from build123d import *

# Parameters (mm, degrees)
SKETCH1_W           = 45
SKETCH1_H           = 187
SKETCH1_R           = 2.2
SKETCH1_R_2         = 2.075
BOSS_EXTRUDE1_DEPTH = 4.75
BOSS_EXTRUDE2_START = -15
SKETCH1_3_R         = 2.075
SKETCH1_3_W         = 2
SKETCH1_3_H         = 171
SKETCH1_3_W_2       = 3
BOSS_EXTRUDE2_DEPTH = 15


with BuildPart() as part:
    # Sketch1 → Boss-Extrude1 (new body)
    with BuildSketch(Plane.XY):
        with Locations((8, 0)):
            Rectangle(SKETCH1_W, SKETCH1_H)
        with Locations((0, -75.75)):
            Circle(SKETCH1_R, mode=Mode.SUBTRACT)
        with Locations((16, -75.75)):
            Circle(SKETCH1_R, mode=Mode.SUBTRACT)
        with Locations((0, 75.75)):
            Circle(SKETCH1_R, mode=Mode.SUBTRACT)
        with Locations((16, 75.75)):
            Circle(SKETCH1_R, mode=Mode.SUBTRACT)
        with Locations((8, -89.5)):
            Circle(SKETCH1_R_2, mode=Mode.SUBTRACT)
        with Locations(Location((8, 89.5, 0), (0, 0, 180))):
            Circle(SKETCH1_R_2, mode=Mode.SUBTRACT)
    extrude(amount=BOSS_EXTRUDE1_DEPTH)

    # Sketch1<3> → Boss-Extrude2 (add)
    # profile 1 of 5: a face of its own
    with BuildSketch(Plane.XY.offset(BOSS_EXTRUDE2_START)):
        Polygon((-12.5, 85.5), (-6.5, 85.5), (6.5, 85.5), (9.5, 85.5), (22.5, 85.5), (28.5, 85.5), (30.5, 85.5), (30.5, 93.5), (-14.5, 93.5), (-14.5, 85.5), align=None)
        with Locations(Location((8, 89.5, 0), (0, 0, 180))):
            Circle(SKETCH1_3_R, mode=Mode.SUBTRACT)
    # profile 2 of 5: a face of its own
    with BuildSketch(Plane.XY.offset(BOSS_EXTRUDE2_START)):
        with Locations((-13.5, 0)):
            Rectangle(SKETCH1_3_W, SKETCH1_3_H)
    # profile 3 of 5: a face of its own
    with BuildSketch(Plane.XY.offset(BOSS_EXTRUDE2_START)):
        Polygon((6.5, -85.5), (-6.5, -85.5), (-12.5, -85.5), (-14.5, -85.5), (-14.5, -93.5), (30.5, -93.5), (30.5, -85.5), (28.5, -85.5), (22.5, -85.5), (9.5, -85.5), align=None)
        with Locations(Location((8, -89.5, 0), (0, 0, 270))):
            Circle(SKETCH1_3_R, mode=Mode.SUBTRACT)
    # profile 4 of 5: a face of its own
    with BuildSketch(Plane.XY.offset(BOSS_EXTRUDE2_START)):
        with Locations((29.5, 0)):
            Rectangle(SKETCH1_3_W, SKETCH1_3_H)
    # profile 5 of 5: a face of its own
    with BuildSketch(Plane.XY.offset(BOSS_EXTRUDE2_START)):
        with Locations((8, 0)):
            Rectangle(SKETCH1_3_W_2, SKETCH1_3_H)
    extrude(amount=BOSS_EXTRUDE2_DEPTH)


solid = part.part
Here's how the part is built. I have some questions about the finished solid (model axes, mm). A direction names the side the tool comes from. Coordinates: 2 decimals unless noted, no trailing zeros. Loops run counter-clockwise (first coordinate to the right, second up) from the corner with the lowest first, then second, coordinate; pieces in that order, holes last.
1. For P1, Ø8, axis at x = 24, y = -32.5, coming from the -Z side; P2, Ø3.5, axis at x = 8, y = -89.5, coming from the -Z side, each with a flat end and sliding along its axis, tell me the tip position at first contact or that it passes through.
2. If we mould it in two halves opening along Y, with no side actions, what happens to faces 3 (the cylindrical face through (9.83, -90.48, -5.26)), 4 (the flat face through (8, -6, -15)), 5 (the cylindrical face through (17.183, -73.895, 2.342)), 6 (the flat face through (8, 93.5, -5))? For each: pulls with the +Y half, pulls with the -Y half, needs draft (parallel to the pull), parting line crosses it, or undercut.
3. Imagine slicing it at A-A, the plane y = 89.5. Please give me the cut outline in (x, z) (3 decimals), and give its area (3 significant figures).
4. I need wall thicknesses on L1, parallel to Y at x = 16, z = 2.95; L2, parallel to X at y = 73.5, z = -1.5; L3, parallel to Y at x = 8, z = -2.5 (3 decimals). Which ranges of each line are inside material? Lowest first, please.
5. Imagine slicing it at C-C, the plane y = -75.75. Please give me the cut outline in (x, z), and give its area (3 significant figures).
6. Imagine slicing it at B-B, the plane x = 0. Please give me the cut outline in (y, z), and give its area (3 significant figures).
7. For faces 1 (the flat face through (6.5, -1, -8)), 2 (the flat face through (30.5, -1, -5)), which set-ups out of +Z, -Z, +X, -X, +Y, -Y let a thin tool reach every point of the face, with its end or its side?
8. Imagine slicing it at D-D, the plane x = -8.5. Please give me the cut outline in (y, z).
Taken from the geometry:
1. P1: stops at z = 0
1. P2: passes through
2. face 3: undercut
2. face 4: needs draft
2. face 5: undercut
2. face 6: pulls with the +Y half
3. outline: (-14.5, -15) - (5.925, -15) - (5.925, 4.75) - (-14.5, 4.75) - close; (10.075, -15) - (30.5, -15) - (30.5, 4.75) - (10.075, 4.75) - close
3. area: 807 mm2
4. L1: y = -93.5 to -77.95, -73.55 to 73.55, 77.95 to 93.5
4. L2: x = -14.5 to -12.5, 6.5 to 9.5, 28.5 to 30.5
4. L3: y = -93.5 to -91.575, -87.425 to 87.425, 91.575 to 93.5
5. outline: (-14.5, -15) - (-12.5, -15) - (-12.5, 0) - (-2.2, 0) - (-2.2, 4.75) - (-14.5, 4.75) - close; (2.2, 0) - (6.5, 0) - (6.5, -15) - (9.5, -15) - (9.5, 0) - (13.8, 0) - (13.8, 4.75) - (2.2, 4.75) - close; (18.2, 0) - (28.5, 0) - (28.5, -15) - (30.5, -15) - (30.5, 4.75) - (18.2, 4.75) - close
5. area: 277 mm2
6. outline: (-93.5, -15) - (-85.5, -15) - (-85.5, 0) - (-77.95, 0) - (-77.95, 4.75) - (-93.5, 4.75) - close; (-73.55, 0) - (73.55, 0) - (73.55, 4.75) - (-73.55, 4.75) - close; (77.95, 0) - (85.5, 0) - (85.5, -15) - (93.5, -15) - (93.5, 4.75) - (77.95, 4.75) - close
6. area: 1,090 mm2
7. face 1: -Z
7. face 2: +Z, -Z, +X, +Y, -Y
8. outline: (-93.5, -15) - (-85.5, -15) - (-85.5, 0) - (85.5, 0) - (85.5, -15) - (93.5, -15) - (93.5, 4.75) - (-93.5, 4.75) - close
